The model under review builds one solid part; all positions refer to its coordinate system, in mm. Face numbers are marked on the shaded views. A direction names the side the tool comes from. Give positions to 0.01 mm unless a question says otherwise; leave off trailing zeros. Loops run counter-clockwise (first coordinate to the right, second up) from the corner with the lowest first, then second, coordinate; pieces in that order, holes last. Notation, with made-up numbers: M 23.5,60.5 L 60.5,60.5 A5 ccw 60.5,67.5 Z; hole C -30,-24 d3. An arc over 180 degrees is marked long. Return JSON: item names as keys, results as strings.
```python
from build123d import *

# Parameters (mm, degrees)
F0_W        = 70.7
F0_H        = 43.1
F3_DEPTH    = 3
F1_R        = 1.6
F4_DEPTH    = 3
F2_W        = 15.5
F2_H        = 14
F2_W_2      = 5.3
F2_H_2      = 4
F2_H_3      = 4.6764186437
F2_W_3      = 21.7
F5_DEPTH    = 3
F6_T1_DEPTH = 27.4948974279
F6_T3_DEPTH = 28
F7_W        = 1
F7_H        = 14
F7_H_2      = 7
F7_W_2      = 15.7
F7_H_3      = 1
F8_DEPTH    = 10


# Not quite as in the source:
# - a fillet or chamfer that OpenCascade refuses, or shapes differently, is made with other operations: its cross-section is extruded or revolved along the edge and cut away or added


with BuildPart() as f3:
    # F0 (on Front) → F3 (new body)
    with BuildSketch(Plane.XZ):
        Rectangle(F0_W, F0_H)
    extrude(amount=F3_DEPTH)

    # F1 (on face) → F4 (cut)
    with BuildSketch(Plane.XZ):
        Polygon((0, -12.0528372875), (0, -18.8028372875), (24, -18.8028372875), (26, -5.3028372875), (0, -5.3028372875), align=None)
        Polygon((-24, -18.8028372875), (0, -18.8028372875), (0, -12.0528372875), (-25, -12.0528372875), align=None)
        with Locations((-29.85, -12.0528372875)):
            Circle(F1_R)
        Polygon((-25, -12.0528372875), (0, -12.0528372875), (0, -5.3028372875), (-26, -5.3028372875), align=None)
        with Locations((29.85, -12.0528372875)):
            Circle(F1_R)
    extrude(amount=F4_DEPTH, mode=Mode.SUBTRACT)

    # F2 (on face) → F5 (cut)
    with BuildSketch(Plane.XZ):
        with Locations((-23.6, 5.1971627125)):
            Rectangle(F2_W, F2_H)
        with Locations((-28.7, 14.8735813563)):
            Rectangle(F2_W_2, F2_H_2)
        with Locations((-28.7, 19.2117906781)):
            Rectangle(F2_W_2, F2_H_3)
        with BuildLine():
            ThreePointArc((-21.675, 16.8735813563), (-17.675, 12.8735813563), (-13.675, 16.8735813563))
            Line((-13.675, 16.8735813563), (-21.675, 16.8735813563))
        make_face()
        with BuildLine():
            Line((-21.675, 16.8735813563), (-13.675, 16.8735813563))
            ThreePointArc((-13.675, 16.8735813563), (-17.675, 20.8735813563), (-21.675, 16.8735813563))
        make_face()
        with BuildLine():
            ThreePointArc((21.675, 16.8735813563), (17.675, 20.8735813563), (13.675, 16.8735813563))
            Line((13.675, 16.8735813563), (21.675, 16.8735813563))
        make_face()
        with BuildLine():
            Line((21.675, 16.8735813563), (13.675, 16.8735813563))
            ThreePointArc((13.675, 16.8735813563), (17.675, 12.8735813563), (21.675, 16.8735813563))
        make_face()
        with BuildLine():
            ThreePointArc((-4, 16.8735813563), (-2.8284271247, 14.0451542315), (0, 12.8735813563))
            Line((0, 12.8735813563), (0, 16.8735813563))
            Line((0, 16.8735813563), (-4, 16.8735813563))
        make_face()
        with BuildLine():
            Line((0, 16.8735813563), (0, 12.8735813563))
            ThreePointArc((0, 12.8735813563), (2.8284271247, 14.0451542315), (4, 16.8735813563))
            Line((4, 16.8735813563), (0, 16.8735813563))
        make_face()
        with Locations((20.5, 5.1971627125)):
            Rectangle(F2_W_3, F2_H)
        Polygon((-10.85, 12.1971627125), (-10.85, -1.8028372875), (4.65, -1.8028372875), (4.65, 12.1971627125), (0, 12.1971627125), align=None)
        with BuildLine():
            Line((-4, 16.8735813563), (0, 16.8735813563))
            Line((0, 16.8735813563), (0, 20.8735813563))
            ThreePointArc((0, 20.8735813563), (-2.8284271247, 19.702008481), (-4, 16.8735813563))
        make_face()
        with BuildLine():
            Line((0, 20.8735813563), (0, 16.8735813563))
            Line((0, 16.8735813563), (4, 16.8735813563))
            ThreePointArc((4, 16.8735813563), (2.8284271247, 19.702008481), (0, 20.8735813563))
        make_face()
    extrude(amount=F5_DEPTH, mode=Mode.SUBTRACT)

    # F6: fillet of radius 5 on 4 edges, made by hand

    # F6_s2 → F6_t1 (cut)
    with BuildSketch(Plane.XZ.offset(-12.2474487139)):
        with BuildLine():
            ThreePointArc((-35.35, 16.6510205144), (-34.2229833462, 19.8132981746), (-31.35, 21.55))
            Line((-31.35, 21.55), (-35.35, 21.55))
            Line((-35.35, 21.55), (-35.35, 16.6510205144))
        make_face()
    extrude(amount=F6_T1_DEPTH, mode=Mode.SUBTRACT)

    # F6_s4 → F6_t3 (cut)
    with BuildSketch(Plane.XZ.offset(-12.5)):
        with BuildLine():
            ThreePointArc((35.35, 16.55), (33.8855339059, 20.0855339059), (30.35, 21.55))
            Line((30.35, 21.55), (35.35, 21.55))
            Line((35.35, 21.55), (35.35, 16.55))
        make_face()
        with BuildLine():
            ThreePointArc((30.35, -21.55), (33.8855339059, -20.0855339059), (35.35, -16.55))
            Line((35.35, -16.55), (35.35, -21.55))
            Line((35.35, -21.55), (30.35, -21.55))
        make_face()
        with BuildLine():
            ThreePointArc((-35.35, -16.55), (-33.8855339059, -20.0855339059), (-30.35, -21.55))
            Line((-30.35, -21.55), (-35.35, -21.55))
            Line((-35.35, -21.55), (-35.35, -16.55))
        make_face()
    extrude(amount=F6_T3_DEPTH, mode=Mode.SUBTRACT)

    # F7 (on face) → F8 (join)
    with BuildSketch(Plane(origin=(0, 0, 0), x_dir=(-1, 0, 0), z_dir=(0, 1, 0))):
        Polygon((15.75, -2.0028372875), (15.75, -3.0028372875), (31.45, -3.0028372875), (31.45, -2.0028372875), (23.6, -2.0028372875), align=None)
        Polygon((31.45, -2.0028372875), (31.45, -3.0028372875), (32.55, -1.8028372875), (31.55, -1.8028372875), align=None)
        with Locations((32.05, 5.1971627125)):
            Rectangle(F7_W, F7_H)
        Polygon((14.65, -1.8028372875), (15.75, -3.0028372875), (15.75, -2.0028372875), (15.65, -1.8028372875), align=None)
        with Locations((15.15, 1.6971627125)):
            Rectangle(F7_W, F7_H_2)
        with Locations((15.15, 8.6971627125)):
            Rectangle(F7_W, F7_H_2)
        with Locations((3.1, -2.5028372875)):
            Rectangle(F7_W_2, F7_H_3)
        Polygon((-5.85, -1.8028372875), (-4.75, -3.0028372875), (-4.75, -2.0028372875), (-4.85, -1.8028372875), align=None)
        with Locations((-5.35, 5.1971627125)):
            Rectangle(F7_W, F7_H)
        with Locations((11.55, 1.6971627125)):
            Rectangle(F7_W, F7_H_2)
        with Locations((11.55, 8.6971627125)):
            Rectangle(F7_W, F7_H_2)
        Polygon((10.95, -3.0028372875), (12.05, -1.8028372875), (11.05, -1.8028372875), (10.95, -2.0028372875), align=None)
    extrude(amount=F8_DEPTH)


solid = f3.part
```
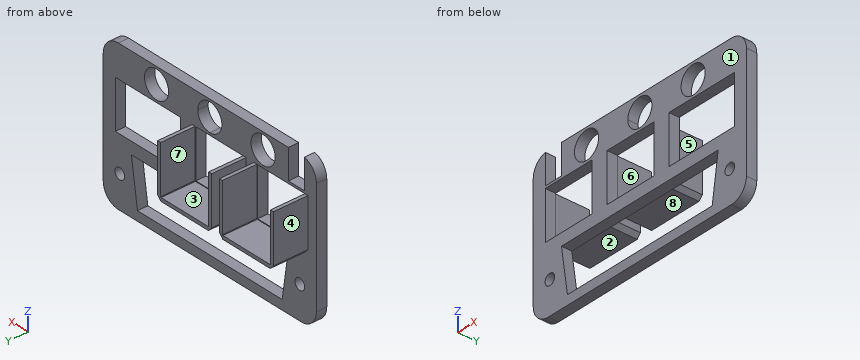
1) Tool access review of the marked faces 1, 2, 3 and 4: name each direction out of +Z, -Z, +X, -X, +Y, -Y from which nothing blocks a thin tool from reaching the whole face with its end or side.
From the geometry:
{"face 1": "+Z, -Z, +X, -X, -Y", "face 2": "-Z, +X, -X, +Y", "face 3": "+Z, +Y", "face 4": "+Z, -Z, -X, +Y"}
2) Insertion check: pin 1 (1.5 mm diameter, centred on y = -1.5, z = 18, fed in from -X); pin 2 (6 mm diameter, centred on x = -24, y = 8, fed in from -Z); pin 3 (4 mm diameter, centred on y = 8.5, z = 7.5, fed in from +X). Each pin has a flat end and moves straight along its axis. Give the tip position at first contact, or say it passes through.
From the geometry:
{"pin 1": "x = -35.31", "pin 2": "z = -3", "pin 3": "x = 5.85"}
3) The part is to be moulded in two halves that separate along X. For the marked faces 5, 6, 7 and 8, say which applies: released by +X, released by -X, zero draft, split by the parting line, or undercut.
From the geometry:
{"face 5": "released by +X", "face 6": "undercut", "face 7": "undercut", "face 8": "zero draft"}
4) Wall thickness on L1, parallel to X at y = 7, z = 10.5; L2, parallel to Z at x = 29.85, y = -0.85; L3, parallel to Z at x = -11, y = -2: over which ranges is each line inside the solid? List them lowest first. Write a range as from..to.
From the geometry:
{"L1": "-32.55..-31.55, -15.65..-14.65, -12.05..-11.05, 4.85..5.85", "L2": "-21.55..-13.65, -10.45..-1.8, 12.2..21.55", "L3": "-21.55..-18.8, -5.3..21.55"}
5) Consider section B-B on z = 0. Count the separate pieces of the cut face and the enclosed holes in it, then the cut area to 3 significant figures.
From the geometry:
{"separate pieces": "4", "enclosed holes": "0", "area": "94.0 mm²"}
6) Consider section A-A on y = 1.25. Write out the cut boundary in (x, z).
From the geometry:
{"outline": "M -32.55,-1.8 L -31.45,-3 L -15.75,-3 L -14.65,-1.8 L -14.65,12.2 L -15.65,12.2 L -15.65,-1.8 L -15.75,-2 L -31.45,-2 L -31.55,-1.8 L -31.55,12.2 L -32.55,12.2 Z; M -12.05,-1.8 L -10.95,-3 L 4.75,-3 L 5.85,-1.8 L 5.85,12.2 L 4.85,12.2 L 4.85,-1.8 L 4.75,-2 L -10.95,-2 L -11.05,-1.8 L -11.05,12.2 L -12.05,12.2 Z"}
7) Consider section C-C on x = -27. Write out the cut boundary in (y, z).
From the geometry:
{"outline": "M -3,-21.55 L 0,-21.55 L 0,-3 L 10,-3 L 10,-2 L 0,-2 L 0,-1.8 L -3,-1.8 Z; M -3,12.2 L 0,12.2 L 0,12.87 L -3,12.87 Z"}
8) Consider section D-D on z = 19. Write out the cut boundary in (x, y), then the cut area to 3 significant figures.
From the geometry:
{"outline": "M -34.76,-3 L -31.35,-3 L -31.35,0 L -34.76,0 Z; M -26.05,-3 L -21.06,-3 L -21.06,0 L -26.05,0 Z; M -14.29,-3 L -3.39,-3 L -3.39,0 L -14.29,0 Z; M 3.39,-3 L 14.29,-3 L 14.29,0 L 3.39,0 Z; M 21.06,-3 L 34.71,-3 L 34.71,0 L 21.06,0 Z", "area": "132 mm²"}
